The listing builds one solid part. Answer for the finished solid, in the listing's coordinates (mm). A direction names the side the tool comes from. Round coordinates to 2 decimals unless told otherwise and drop trailing zeros. Order: outer loops, then holes, each group sorted by start corner. A loop starts at its lowest first (then second) coordinate and runs counter-clockwise, first axis right, second up. Notation, with made-up numbers: M 64.25,79 L 76.25,79 A13 ccw 76.25,88 Z; hole C -3.75,69.5 d11. An arc over 180 degrees is marked long. Put each result on its own line as item: value. Start each with the question number.
1. Consider line 1 (Z direction, x = -3.25, y = -3); line 2 (X direction, y = -8.5, z = 2.25); line 3 (Y direction, x = -5.5, z = 0.3). Determine where each line is inside the solid, lowest interval first.
2. The part is cut by section D-D (x = -3.5). Give the vertices of the cut face in (y, z), then the cut area to 3 significant figures.
3. The part is cut by section B-B (x = 4). Give the vertices of the cut face in (y, z).
4. The part is cut by section A-A (y = -12). Give the vertices of the cut face in (x, z).
5. Which of the six approach directions +Z, -Z, +X, -X, +Y, -Y give full straight-line access (tool end or side, diameter ignored) to faces 1 (the face through (5.2, -20.3, 0.5)), 2 (the face through (2.2, -11, 3)), 3 (the face through (4, -15.8, 2.8)), 4 (the face through (5.8, -11, 3)), 5 (the face through (-5.3, -20.3, 0.5))?
6. Each of these flat-tipped pins is pushed along its axis until it touches: pin 1 Ø0.6 at (x, z) = (7, 0.5) entering from -Y; pin 2 Ø2 at (y, z) = (-15, 3) entering from -X; pin 3 Ø0.6 at (y, z) = (-21, 1) entering from -X. Where does it stop, or does it pass through?
7. The part is cut by section C-C (z = 0.5). Give the vertices of the cut face in (x, y).
from build123d import *

# Parameters (mm, degrees)
SKETCH_1_W      = 20.6
SKETCH_1_H      = 40.6
EXTRUDE_1_DEPTH = 1.1
EXTRUDE_2_DEPTH = 3.5
SKETCH_3_W      = 1.46922728
SKETCH_3_H      = 3.03026103
EXTRUDE_3_DEPTH = 1.1
CHAMFER_1_SIZE  = 0.5


with BuildPart() as part:
    # Эскиз1 → Бобышка-Вытянуть1 (new body)
    with BuildSketch(Plane.XY):
        Rectangle(SKETCH_1_W, SKETCH_1_H)
    extrude(amount=EXTRUDE_1_DEPTH)

    # Эскиз2 → Бобышка-Вытянуть2 (add)
    with BuildSketch(Plane.XY.offset(1.1)):
        with BuildLine():
            Line((5.8, -7.6), (5.8, -14))
            ThreePointArc((5.8, -14), (4, -15.8), (2.2, -14))
            Line((2.2, -14), (2.2, -7.6))
            ThreePointArc((2.2, -7.6), (4, -5.8), (5.8, -7.6))
        make_face()
    extrude(amount=EXTRUDE_2_DEPTH)

    # Эскиз3 → Бобышка-Вытянуть3 (add)
    with BuildSketch(Plane.XY.offset(1.1)):
        with Locations((0, -20.3)):
            Rectangle(SKETCH_3_W, SKETCH_3_H)
    extrude(amount=-EXTRUDE_3_DEPTH)

    # Фаска1
    chamfer_1_edges = [part.edges().sort_by_distance(p)[0] for p in [
        (10.3, -20.3, 0.55),
        (-10.3, -20.3, 0.55),
        (-10.3, 20.3, 0.55),
        (10.3, 20.3, 0.55),
    ]]
    chamfer(chamfer_1_edges, length=CHAMFER_1_SIZE)


solid = part.part
Resolved:
1. line 1: 0 to 1.1
1. line 2: 2.2 to 5.8
1. line 3: -20.3 to 20.3
2. outline: M -20.3,0 L 20.3,0 L 20.3,1.1 L -20.3,1.1 Z
2. area: 44.7 mm2
3. outline: M -20.3,0 L 20.3,0 L 20.3,1.1 L -5.8,1.1 L -5.8,4.6 L -15.8,4.6 L -15.8,1.1 L -20.3,1.1 Z
4. outline: M -10.3,0 L 10.3,0 L 10.3,1.1 L 5.8,1.1 L 5.8,4.6 L 2.2,4.6 L 2.2,1.1 L -10.3,1.1 Z
5. face 1: +Z, -Z, +X, -Y
5. face 2: +Z, -X, +Y, -Y
5. face 3: +Z, -Y
5. face 4: +Z, +X, +Y, -Y
5. face 5: +Z, -Z, -X, -Y
6. pin 1: y = -20.3
6. pin 2: x = 2.2
6. pin 3: x = -0.73
7. outline: M -10.3,-19.8 L -9.8,-20.3 L -0.73,-20.3 L -0.73,-21.82 L 0.73,-21.82 L 0.73,-20.3 L 9.8,-20.3 L 10.3,-19.8 L 10.3,19.8 L 9.8,20.3 L -9.8,20.3 L -10.3,19.8 Z
